Can you work these out from the model? Positions are in its coordinate system, mm. A direction names the side the tool comes from. Give positions to 0.01 mm unless a question says otherwise; leave off trailing zeros. Write each loop counter-clockwise with the first axis right and the second up, starting at its lowest first coordinate (ties: lowest second). Pieces come first, ordered by that corner, then holes. Notation, with made-up numbers: M 23.25,-23.75 L 47.25,-23.75 A6 ccw 47.25,-13.75 Z; hole C 14,84.25 d4. An arc over 180 degrees is marked long. Write each question's results on one line, items separated by ' | '.
from build123d import *

# Parameters (mm, degrees)
F0_W           = 80
F0_H           = 80
F1_DEPTH       = 10
F3_D           = 3.3
F3_CSINK_D     = 6.72
F3_CSINK_ANGLE = 90
F2_R           = 11
F4_DEPTH       = 10.001
F5_R           = 9
F6_DEPTH       = 10.001
F7_R           = 11
F8_DEPTH       = 7


with BuildPart() as f1:
    # F0 (on Front) → F1 (new body)
    with BuildSketch(Plane.XZ):
        Rectangle(F0_W, F0_H)
    extrude(amount=F1_DEPTH)

    # F3 (through all)
    with Locations(Plane.XZ.offset(10)):
        with Locations((-33, 33), (-7, 33), (-33, 7)):
            CounterSinkHole(F3_D / 2, F3_CSINK_D / 2, counter_sink_angle=F3_CSINK_ANGLE)

    # F2 (on face) → F4 (cut, through all)
    with BuildSketch(Plane.XZ.offset(10)):
        with Locations((-20, 20)):
            Circle(F2_R)
    extrude(amount=-F4_DEPTH, mode=Mode.SUBTRACT)

    # F5 (on face) → F6 (cut, through all)
    with BuildSketch(Plane.XZ.offset(10)):
        Circle(F5_R)
    extrude(amount=-F6_DEPTH, mode=Mode.SUBTRACT)

    # F7 (on face) → F8 (cut)
    with BuildSketch(Plane.XZ.offset(10)):
        Circle(F7_R)
    extrude(amount=-F8_DEPTH, mode=Mode.SUBTRACT)


solid = f1.part
Item 1: I want a section at B-B, the plane z = 33. Please give me the cut outline in (x, y).
Geometry says:
outline: M -40,-10 L -36.36,-10 L -34.65,-8.29 L -34.65,0 L -40,0 Z; M -31.35,-8.29 L -29.64,-10 L -10.36,-10 L -8.65,-8.29 L -8.65,0 L -31.35,0 Z; M -5.35,-8.29 L -3.64,-10 L 40,-10 L 40,0 L -5.35,0 Z
Item 2: Thinking about a two-plate mould opening in Z: for faces 3 (the face through (-0.6, 0, 9.4)), 4 (the face through (-6.785, -4.087, 34.636)), 5 (the face through (-1, -5, -40)), which applies, +Z half, -Z half, draft (parallel to the pull), parting line (faces both ways), or undercut?
Geometry says:
face 3: draft | face 4: undercut | face 5: -Z half
Item 3: I'm going to push flat-ended pins straight in: pin 1 (17.5 mm diameter, centred on x = 0, z = -0.5, fed in from -Y); pin 2 (5.5 mm diameter, centred on x = -33, z = 33, fed in from -Y); pin 3 (2 mm diameter, centred on x = -33, z = 7, fed in from +Y); pin 4 (1 mm diameter, centred on x = -5.5, z = 31.5, fed in from -Y). Where does each tip first touch, or does it pass through?
Geometry says:
pin 1: stops at y = -3 | pin 2: stops at y = -9.39 | pin 3: passes through | pin 4: stops at y = -9.26
Item 4: For faces 1 (the face through (2, -3, -9)), 2 (the face through (8, -10, -8)), which set-ups out of +Z, -Z, +X, -X, +Y, -Y let a thin tool reach every point of the face, with its end or its side?
Geometry says:
face 1: -Y | face 2: +Z, -Z, +X, -X, -Y
Item 5: I want a section at D-D, the plane y = -4.25. Please give me the cut outline in (x, z), and give its area (3 significant figures).
Geometry says:
outline: M -40,-40 L 40,-40 L 40,40 L -40,40 Z; hole C -33,7 d3.3; hole C -33,33 d3.3; hole C -20,20 d22; hole C 0,0 d22; hole C -7,33 d3.3 | area: 5,610 mm2
Item 6: I want a section at C-C, the plane x = -33. Please give me the cut outline in (y, z), and give its area (3 significant figures).
Geometry says:
outline: M -10,-40 L 0,-40 L 0,5.35 L -8.29,5.35 L -10,3.64 Z; M -10,10.36 L -8.29,8.65 L 0,8.65 L 0,31.35 L -8.29,31.35 L -10,29.64 Z; M -10,36.36 L -8.29,34.65 L 0,34.65 L 0,40 L -10,40 Z | area: 728 mm2
Item 7: I want a section at A-A, the plane z = 20. Please give me the cut outline in (x, y), and give its area (3 significant figures).
Geometry says:
outline: M -40,-10 L -31,-10 L -31,0 L -40,0 Z; M -9,-10 L 40,-10 L 40,0 L -9,0 Z | area: 580 mm2
Item 8: If I drill on line 1 (X direction, y = -3, z = 33); line 2 (Z direction, x = -33, y = -4.75); line 3 (Z direction, x = -20, y = -5), over which ranges is the centre line in solid material (lowest first)? Write a range as from..to.
Geometry says:
line 1: x = -40..-34.65, -31.35..-8.65, -5.35..40 | line 2: z = -40..5.35, 8.65..31.35, 34.65..40 | line 3: z = -40..9, 31..40
